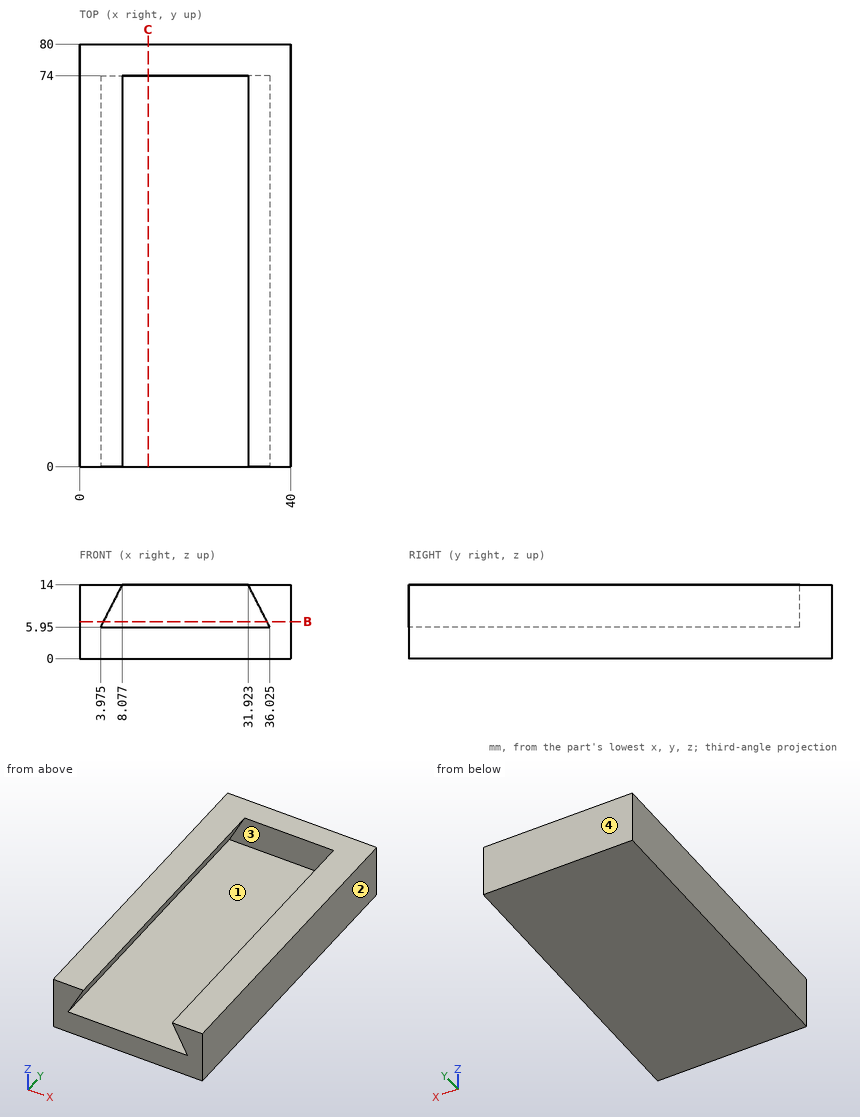
The figure shows three views and two pictorial views of one solid part (mm, origin at its lowest corner). Answer the questions. Coordinates: 2 decimals unless noted, no trailing zeros. Write each loop counter-clockwise with the first axis right and the second up, starting at its lowest first coordinate (ties: lowest second). Pieces come first, ordered by that corner, then holes. Notation, with made-up numbers: (62, -8.75) -> (107, -8.75) arc R28 ccw to (107, 30.25) -> close; hole circle Ø3 at (45, 35). An arc over 180 degrees is marked (long way). Answer as a JSON object with one key per item and string values.
Q1. The part is cut by section B-B on z = 7. Give the vertices of the cut face in (x, y).
The answers:
{"outline": "(0, 0) -> (4.51, 0) -> (4.51, 74) -> (35.49, 74) -> (35.49, 0) -> (40, 0) -> (40, 80) -> (0, 80) -> close"}
Q2. Determine the mould class of the marked faces 1, 2, 3 and 4 for opening direction X: pulls with the +X half, pulls with the -X half, needs draft (parallel to the pull), parting line crosses it, or undercut.
The answers:
{"face 1": "undercut", "face 2": "pulls with the +X half", "face 3": "undercut", "face 4": "needs draft"}
Q3. Consider line 1 (Z direction, x = 23, y = 51.5); line 2 (X direction, y = 48.5, z = 9.25); line 3 (Y direction, x = 20, z = 6). Determine where each line is inside the solid, lowest interval first. Write a range as [from, to].
The answers:
{"line 1": "z = [0, 5.95]", "line 2": "x = [0, 5.66], [34.34, 40]", "line 3": "y = [74, 80]"}
Q4. A flat-ended cylindrical pin translates along its axis: pin 1 Ø4 at (x, z) = (25, 8) entering from -Y. Find the tip coordinate at first contact, or state that the pin passes through.
The answers:
{"pin 1": "stops at y = 74"}
Q5. The part is cut by section C-C on x = 13. Give the vertices of the cut face in (y, z), then the cut area to 3 significant figures.
The answers:
{"outline": "(0, 0) -> (80, 0) -> (80, 14) -> (74, 14) -> (74, 5.95) -> (0, 5.95) -> close", "area": "524 mm2"}
